Here's how the part is built. I have some questions about the finished solid (model axes, mm). A direction names the side the tool comes from. Give positions to 0.01 mm unless a question says otherwise; leave off trailing zeros. Loops run counter-clockwise (first coordinate to the right, second up) from the corner with the lowest first, then second, coordinate; pieces in that order, holes last.
Q1. If we section it at A-A (x = 0): Please give me the cut outline in (y, z), plus the area to 3 significant figures.
Q2. For faces 1 (the face through (2, -9, 6)), 2 (the face through (10, 3.2, 6.5)), 3 (the face through (-0.1, -6.2, 8)), which set-ups out of +Z, -Z, +X, -X, +Y, -Y let a thin tool reach every point of the face, with its end or its side?
Q3. I need wall thicknesses on line 1 (Z direction, x = -5, y = -5.75); line 2 (X direction, y = 0.25, z = 8.5); line 3 (Z direction, x = 9, y = -2.5). Which ranges of each line are inside material? Lowest first, please.
Q4. Will these pins go through, and if not, where does the flat tip stop? P1, Ø1.5, axis at y = -5, z = 2.5, coming from the +X side; P2, Ø3, axis at x = -5.5, y = -2.5, coming from the +Z side; P3, Ø1.5, axis at y = -3.5, z = 13, coming from the +X side.
Q5. If we section it at C-C (z = 4.5): Please give me the cut outline in (x, y), plus the area to 3 significant figures.
from build123d import *

# Parameters (mm, degrees)
F0_R     = 8.8
F1_DEPTH = 8
F2_R     = 6
F3_DEPTH = 3
F4_R     = 4.1
F5_DEPTH = 7
F6_R     = 10.5
F6_R_2   = 8.8
F7_DEPTH = 2
F8_R     = 1


with BuildPart() as f1:
    # F0 (on Top) → F1 (new body)
    with BuildSketch(Plane.XY):
        Circle(F0_R)
    extrude(amount=F1_DEPTH)

    # F2 (on face) → F3 (join)
    with BuildSketch(Plane.XY.offset(8)):
        Circle(F2_R)
    extrude(amount=F3_DEPTH)

    # F4 (on face) → F5 (join)
    with BuildSketch(Plane.XY.offset(11)):
        Circle(F4_R)
    extrude(amount=F5_DEPTH)

    # F6 (on face) → F7 (join)
    with BuildSketch(Plane.XY.offset(8)):
        Circle(F6_R)
        Circle(F6_R_2, mode=Mode.SUBTRACT)
    extrude(amount=-F7_DEPTH)

    # F8
    f8_edges = [f1.edges().sort_by_distance(p)[0] for p in [
        (-4.1, 0, 18),
        (-6, 0, 11),
        (-10.5, 0, 8),
        (-8.8, 0, 0),
    ]]
    fillet(f8_edges, radius=F8_R)


solid = f1.part
Check sheet entries:
1. outline: (-10.5, 6) - (-8.8, 6) - (-8.8, 1) arc R1 ccw to (-7.8, 0) - (7.8, 0) arc R1 ccw to (8.8, 1) - (8.8, 6) - (10.5, 6) - (10.5, 7) arc R1 ccw to (9.5, 8) - (6, 8) - (6, 10) arc R1 ccw to (5, 11) - (4.1, 11) - (4.1, 17) arc R1 ccw to (3.1, 18) - (-3.1, 18) arc R1 ccw to (-4.1, 17) - (-4.1, 11) - (-5, 11) arc R1 ccw to (-6, 10) - (-6, 8) - (-9.5, 8) arc R1 ccw to (-10.5, 7) - close
1. area: 239 mm2
2. face 1: -Z
2. face 2: +Z, -Z
2. face 3: +Z
3. line 1: z = 0 to 8
3. line 2: x = -5.99 to 5.99
3. line 3: z = 6 to 8
4. P1: stops at x = 7.71
4. P2: stops at z = 11
4. P3: stops at x = 3.04
5. outline: circle Ø17.6 at (0, 0)
5. area: 243 mm2
